from build123d import *

# Parameters (mm, degrees)
SKETCH1_R              = 3.706733852
BOSS_EXTRUDE1_DEPTH    = 12
F_12_CLEARANCE_HOLE1_D = 6.15
FILLET1_R              = 10
SKETCH6_R              = 8.05
SKETCH6_R_2            = 2.6
CUT_EXTRUDE1_DEPTH     = 5
SKETCH6_2_R            = 2.6
CUT_EXTRUDE2_DEPTH     = 272.271439088


with BuildPart() as part:
    # Sketch1 → Boss-Extrude1 (new body)
    with BuildSketch(Plane.XY.offset(26)):
        with BuildLine():
            Line((48.415563176, 256.476121426), (23.233399504, 237.5))
            Line((23.233399504, 237.5), (-40, 237.5))
            Line((-40, 237.5), (-40, 162))
            Line((-40, 162), (40, 162))
            Line((40, 162), (40, 206.309791675))
            Line((40, 206.309791675), (69.479088987, 228.523878574))
            ThreePointArc((69.479088987, 228.523878574), (72.923447507, 253.031762905), (48.415563176, 256.476121426))
        make_face()
        with Locations((0, 189)):
            Circle(SKETCH1_R, mode=Mode.SUBTRACT)
    extrude(amount=-BOSS_EXTRUDE1_DEPTH)

    # #12 Clearance Hole1 (through all)
    with Locations(Plane.XY.offset(26)):
        with Locations((31, 172.8), (-31, 205.2), (-31, 172.8), (31, 205.2)):
            Hole(F_12_CLEARANCE_HOLE1_D / 2)

    # Fillet1
    fillet1_edges = [part.edges().sort_by_distance(p)[0] for p in [
        (40, 206.309791675, 20),
        (40, 162, 20),
        (-40, 162, 20),
        (-40, 237.5, 20),
        (23.233399504, 237.5, 20),
    ]]
    fillet(fillet1_edges, radius=FILLET1_R)

    # Sketch6 → Cut-Extrude1 (cut)
    with BuildSketch(Plane.XY.offset(26)):
        with Locations((59.857743265, 243.186048556)):
            Circle(SKETCH6_R)
        with Locations((59.857743265, 243.186048556)):
            Circle(SKETCH6_R_2, mode=Mode.SUBTRACT)
    extrude(amount=-CUT_EXTRUDE1_DEPTH, mode=Mode.SUBTRACT)

    # Sketch6<2> → Cut-Extrude2 (cut, through all)
    with BuildSketch(Plane.XY.offset(26)):
        with Locations((59.857743265, 243.186048556)):
            Circle(SKETCH6_2_R)
    extrude(amount=-CUT_EXTRUDE2_DEPTH, mode=Mode.SUBTRACT)


solid = part.part
CAD build for the part. Positions are in the model's coordinates, mm. A direction names the side the tool comes from. Give positions to 0.01 mm unless a question says otherwise; leave off trailing zeros. Write each loop counter-clockwise with the first axis right and the second up, starting at its lowest first coordinate (ties: lowest second). Pieces come first, ordered by that corner, then holes. Notation, with made-up numbers: M 77,-10.75 L 135,-10.75 A15 ccw 135,6.25 Z; hole C -35.5,-23.5 d1. An arc over 180 degrees is marked long. Put each result on its own line as item: value. Start each with the question number.
(1) Mould opens along X. For faces 4 (the face through (31.4, 208.25, 19.92)), 5 (the face through (41.08, 205.84, 19.92)), 6 (the face through (73.152, 252.722, 20.084)) say: +X half, -X half, draft (parallel to the pull), parting line (faces both ways), or undercut.
(2) Which spindle directions (+Z, -Z, +X, -X, +Y, -Y) get a long thin tool onto all of the face, cutting with end or side? Do faces 1 (the face through (64.19, 249.97, 23.54)), 2 (the face through (-36.99, 234.65, 19.92)), 3 (the face through (40, 186, 20)). Say none if no direction does.
(3) Band-saw the part on D-D, the plane x = 32.5. Write the cut outline in (y, z), and give its area (3 significant figures).
(4) Band-saw the part on C-C, the plane y = 205.2. Write the cut outline in (x, z) (3 decimals).
(5) Flat gauge pins, fed straight in: pin 1 Ø4 at (y, z) = (246, 24.5) entering from +X; pin 2 Ø6.5 at (x, y) = (0, 189) entering from +Z; pin 3 Ø6 at (y, z) = (192, 17.5) entering from +X; pin 4 Ø6 at (x, y) = (59.86, 243.19) entering from +Z. Where does each tip first touch, or does it go through?
(6) Band-saw the part on A-A, the plane x = 0. Write the cut outline in (y, z), and give its area (3 significant figures).
(7) Band-saw the part on B-B, the plane y = 189. Write the cut outline in (x, z), and give its area (3 significant figures).
(8) Probe L1, parallel to X at y = 172.8, z = 23 (3 decimals); L2, parallel to X at y = 206, z = 15.5; L3, parallel to Y at x = 0, z = 17. List the from-to ranges inside material, lowest first.
Response values:
1. face 4: undercut
1. face 5: +X half
1. face 6: parting line
2. face 1: +Z
2. face 2: +Z, -Z, -X, +Y
2. face 3: +Z, -Z, +X, -Y
3. outline: M 162.32,14 L 170.12,14 L 170.12,26 L 162.32,26 Z; M 175.48,14 L 202.52,14 L 202.52,26 L 175.48,26 Z; M 207.88,14 L 244.48,14 L 244.48,26 L 207.88,26 Z
3. area: 857 mm2
4. outline: M -40,14 L -34.075,14 L -34.075,26 L -40,26 Z; M -27.925,14 L 27.925,14 L 27.925,26 L -27.925,26 Z; M 34.075,14 L 40.782,14 L 40.782,26 L 34.075,26 Z
5. pin 1: stops at x = 76.38
5. pin 2: passes through
5. pin 3: stops at x = 40
5. pin 4: stops at z = 21
6. outline: M 162,14 L 185.29,14 L 185.29,26 L 162,26 Z; M 192.71,14 L 237.5,14 L 237.5,26 L 192.71,26 Z
6. area: 817 mm2
7. outline: M -40,14 L -3.71,14 L -3.71,26 L -40,26 Z; M 3.71,14 L 40,14 L 40,26 L 3.71,26 Z
7. area: 871 mm2
8. L1: x = -40 to -34.075, -27.925 to 27.925, 34.075 to 40
8. L2: x = -40 to -33.97, -28.03 to 28.03, 33.97 to 41.16
8. L3: y = 162 to 185.29, 192.71 to 237.5
